The model under review builds one solid part; all positions refer to its coordinate system, in mm. Face numbers are marked on the shaded views. A direction names the side the tool comes from. Round coordinates to 2 decimals unless told otherwise and drop trailing zeros. Write each loop counter-clockwise with the first axis right and the second up, starting at its lowest first coordinate (ties: lowest second). Pieces come first, ordered by that corner, then holes. Notation, with made-up numbers: M 68,16.25 L 118,16.25 A24 cw 118,33.25 Z; hole C -9.5,83.25 d3. An arc over 180 degrees is marked long. One line per item, written item: value. Start each with the question number.
1) Take a section at A-A, the plane z = 2. Write out the cut boundary in (x, y), and give its area (3 significant figures).
2) For P1, Ø2, axis at x = 32, y = 10.5, coming from the -Z side; P2, Ø6, axis at x = 19, z = 9, coming from the -Y side; P3, Ø6, axis at y = 6.5, z = 5.5, coming from the -X side; P4, Ø6, axis at x = 13, y = 1, coming from the -Z side, all flat-tipped, find the tip position at first contact; note any pin that passes through.
3) Mouldability with a two-part tool opening along X and no side actions: class the marked faces 1, 2 and 3 as +X half, -X half, draft (parallel to the pull), parting line (faces both ways), or undercut.
4) Take a section at B-B, the plane y = 3.75. Write out the cut boundary in (x, z), and give its area (3 significant figures).
5) Take a section at C-C, the plane z = 11. Write out the cut boundary in (x, y), and give its area (3 significant figures).
6) Take a section at D-D, the plane x = 25.5. Write out the cut boundary in (y, z).
7) Tool access review of the marked faces 4, 5 and 6: name each direction out of +Z, -Z, +X, -X, +Y, -Y from which nothing blocks a thin tool from reaching the whole face with its end or side.
8) Wall thickness on probe 1 along Y at (x, z) = (18.5, 6.25); probe 2 along X at (y, z) = (5.5, 8); probe 3 along Z at (x, y) = (39, 18): over which ranges is each line inside the solid? List them lowest first.
from build123d import *

# Parameters (mm, degrees)
SKETCH001_W  = 44
SKETCH001_H  = 24
PAD_DEPTH    = 12
BOX_W        = 12
BOX_H        = 2
BOX_DEPTH    = 12
BOX001_W     = 40.2
BOX001_H     = 20.2
BOX001_DEPTH = 10


with BuildPart() as part:
    # Sketch001 → Pad (new body)
    with BuildSketch(Plane.XY):
        with Locations((20, 10)):
            Rectangle(SKETCH001_W, SKETCH001_H)
    extrude(amount=PAD_DEPTH)

    # Box → Box (join)
    with BuildSketch(Plane(origin=(-1, 0, 0), x_dir=(-0.866025, -0.5, 0), z_dir=(0, 0, 1))):
        with Locations((6, 1)):
            Rectangle(BOX_W, BOX_H)
    extrude(amount=BOX_DEPTH)

    # Box001 → Box001 (cut)
    with BuildSketch(Plane(origin=(-0.1, -0.1, 0), x_dir=(1, 0, 0), z_dir=(0, 0, 1))):
        with Locations((20.1, 10.1)):
            Rectangle(BOX001_W, BOX001_H)
    extrude(amount=BOX001_DEPTH, mode=Mode.SUBTRACT)

    # Cone → Cone (revolve, cut)
    with BuildSketch(Plane(origin=(-5, -2, 6), x_dir=(0.866025, 0.5, 0), z_dir=(0, 0, -1))):
        Polygon((0, 0), (2, 0), (3, 2.5), (0, 2.5), align=None)
    revolve(axis=Axis((-5, -2, 6), (0.5, -0.866025, 0)), mode=Mode.SUBTRACT)

    # Cone001 → Cone001 (revolve, cut)
    with BuildSketch(Plane(origin=(-4, -4, 6), x_dir=(-0.866025, -0.5, 0), z_dir=(0, 0, -1))):
        Polygon((0, 0), (2, 0), (3, 2.5), (0, 2.5), align=None)
    revolve(axis=Axis((-4, -4, 6), (-0.5, 0.866025, 0)), mode=Mode.SUBTRACT)


solid = part.part
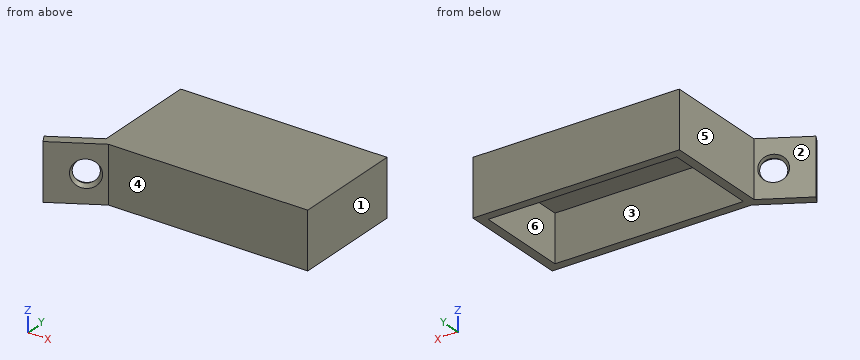
Checked values:
1. outline: M -11.39,-6 L -10.39,-7.73 L -0.46,-2 L 42,-2 L 42,22 L -2,22 L -2,-0.58 Z; hole M -0.1,-0.1 L 40.1,-0.1 L 40.1,20.1 L -0.1,20.1 Z
1. area: 265 mm2
2. P1: stops at z = 10
2. P2: stops at y = -2
2. P3: stops at x = -2
2. P4: stops at z = 0
3. face 1: +X half
3. face 2: -X half
3. face 3: undercut
4. outline: M -2,0 L -0.1,0 L -0.1,10 L 40.1,10 L 40.1,0 L 42,0 L 42,12 L -2,12 Z
4. area: 126 mm2
5. outline: M -11.39,-6 L -10.39,-7.73 L -0.46,-2 L 42,-2 L 42,22 L -2,22 L -2,-0.58 Z
5. area: 1,080 mm2
6. outline: M -2,0 L -0.1,0 L -0.1,10 L 20.1,10 L 20.1,0 L 22,0 L 22,12 L -2,12 Z
7. face 4: +Z, -Z, +X, -Y
7. face 5: +Z, -Z, -X, +Y
7. face 6: -Z
8. probe 1: y = -2 to -0.1, 20.1 to 22
8. probe 2: x = -2 to -0.1, 40.1 to 42
8. probe 3: z = 10 to 12
